from build123d import *

# Parameters (mm, degrees)
F1_DEPTH  = 30
F3_DEPTH  = 100
F4_R      = 50
F5_W      = 30
F5_H      = 30
F6_DEPTH  = 865
F8_W      = 1500
F8_H      = 460
F9_DEPTH  = 30
F11_W     = 780
F11_H     = 320
F12_DEPTH = 30
F13_W     = 30
F13_H     = 30
F14_DEPTH = 220
F15_W     = 30
F15_H     = 30
F16_DEPTH = 260
F17_W     = 780
F17_H     = 2
F18_DEPTH = 50
F19_R     = 20


with BuildPart() as f1:
    # F0 (on Top) → F1 (new body)
    with BuildSketch(Plane.XY):
        Polygon((0, 520), (0, 0), (1650, 0), (1650, 290), (1580, 290), (1580, 590), (150, 590), (150, 520), align=None)
    extrude(amount=F1_DEPTH)

    # F2 (on face) → F3 (join)
    with BuildSketch(Plane.XY.offset(30)):
        Polygon((1648, 0), (1650, 0), (1650, 290), (1580, 290), (1580, 590), (150, 590), (150, 520), (0, 520), (0, 518), (152, 518), (152, 588), (1578, 588), (1578, 288), (1648, 288), align=None)
    extrude(amount=F3_DEPTH)

    # F4
    f4_edges = [f1.edges().sort_by_distance(p)[0] for p in [
        (0, 519, 130),
        (1649, 0, 130),
    ]]
    fillet(f4_edges, radius=F4_R)

    # F5 (on face) → F6 (join)
    with BuildSketch(Plane(origin=(0, 0, 0), x_dir=(1, 0, 0), z_dir=(0, 0, -1))):
        with Locations((65, -45)):
            Rectangle(F5_W, F5_H)
        with Locations((1535, -45)):
            Rectangle(F5_W, F5_H)
        with Locations((1535, -475)):
            Rectangle(F5_W, F5_H)
        with Locations((65, -475)):
            Rectangle(F5_W, F5_H)
    extrude(amount=F6_DEPTH)

    # F8 (on offset) → F9 (join)
    with BuildSketch(Plane(origin=(0, 0, -715), x_dir=(1, 0, 0), z_dir=(0, 0, -1))):
        with Locations((800, -260)):
            Rectangle(F8_W, F8_H)
    extrude(amount=F9_DEPTH)



with BuildPart() as f12:
    # F11 (on offset) → F12 (new body)
    with BuildSketch(Plane.XY.offset(280)):
        with Locations((440, 185)):
            Rectangle(F11_W, F11_H)
    extrude(amount=-F12_DEPTH)


with BuildPart() as f1_1:
    add(f1.part)

    add(f12.part)  # F14 merges F12
    # F13 (on face) → F14 (join, through all)
    with BuildSketch(Plane(origin=(0, 0, 250), x_dir=(1, 0, 0), z_dir=(0, 0, -1))):
        with Locations((65, -40)):
            Rectangle(F13_W, F13_H)
        with Locations((65, -330)):
            Rectangle(F13_W, F13_H)
        with Locations((815, -40)):
            Rectangle(F13_W, F13_H)
        with Locations((815, -330)):
            Rectangle(F13_W, F13_H)
    extrude(amount=F14_DEPTH)

    # F15 (on face) → F16 (join, through all)
    with BuildSketch(Plane.XZ.offset(-315)):
        with Locations((65, 45)):
            Rectangle(F15_W, F15_H)
        with Locations((815, 45)):
            Rectangle(F15_W, F15_H)
    extrude(amount=F16_DEPTH)

    # F17 (on face) → F18 (join)
    with BuildSketch(Plane.XY.offset(280)):
        with Locations((440, 344)):
            Rectangle(F17_W, F17_H)
    extrude(amount=F18_DEPTH)

    # F19
    f19_edges = [f1_1.edges().sort_by_distance(p)[0] for p in [
        (50, 344, 330),
        (830, 344, 330),
    ]]
    fillet(f19_edges, radius=F19_R)


solid = f1_1.part
Check sheet for the modelled part. Datum: model origin and axes. Units: mm. A direction names the side the tool comes from. Round coordinates to 2 decimals unless told otherwise and drop trailing zeros. Loops run counter-clockwise (first coordinate to the right, second up) from the corner with the lowest first, then second, coordinate; pieces in that order, holes last. Notation, with made-up numbers: M -31,-36 L -17,-36 A21 ccw -17,-30 Z; hole C 24,17 d2. An arc over 180 degrees is marked long. One line per item, written item: value.
(1) Thickness scan on line 1 (Z direction, x = 471, y = 202); line 2 (X direction, y = 47.5, z = -491.5); line 3 (Z direction, x = 484, y = 407). Record the ranges inside material, lowest first.
Computed values:
line 1: z = -745 to -715, 0 to 30, 250 to 280
line 2: x = 50 to 80, 1520 to 1550
line 3: z = -745 to -715, 0 to 30
(2) Sectioned sample at B-B, the plane x = 1276.5. Record the cut outline in (y, z).
Computed values:
outline: M 0,0 L 590,0 L 590,130 L 588,130 L 588,30 L 0,30 Z; M 30,-745 L 490,-745 L 490,-715 L 30,-715 Z
(3) Sectioned sample at D-D, the plane x = 294. Record the cut outline in (y, z).
Computed values:
outline: M 0,0 L 590,0 L 590,130 L 588,130 L 588,30 L 0,30 Z; M 25,250 L 345,250 L 345,330 L 343,330 L 343,280 L 25,280 Z; M 30,-745 L 490,-745 L 490,-715 L 30,-715 Z
(4) Access from +Z, -Z, +X, -X, +Y, -Y to the whole of each face (thin tool, end or side, straight path). Record for faces 4 (the face through (1648, 146, 79)), 5 (the face through (438, 25, 257)), 6 (the face through (75, 518, 79)).
Computed values:
face 4: +Z, -Y
face 5: +Z, -X, -Y
face 6: +Z, -X
(5) Release check for a two-part mould opening along X. For faces 1 (the face through (76, 520, 64)), 2 (the face through (800, 186, 59)), 3 (the face through (50, 466, -463)) record: +X half, -X half, draft (parallel to the pull), parting line (faces both ways), or undercut.
Computed values:
face 1: draft
face 2: undercut
face 3: -X half
(6) Sectioned sample at A-A, the plane z = 188.5. Record the cut outline in (x, y).
Computed values:
outline: M 50,25 L 80,25 L 80,55 L 50,55 Z; M 50,315 L 80,315 L 80,345 L 50,345 Z; M 800,25 L 830,25 L 830,55 L 800,55 Z; M 800,315 L 830,315 L 830,345 L 800,345 Z
(7) Depth check by flat-ended pin: pin 1 Ø1.5 at (x, z) = (349, -728) entering from -Y; pin 2 Ø15 at (x, y) = (820.5, 136) entering from +Z; pin 3 Ø8 at (x, y) = (1228, 100.5) entering from +Z. Enter the tip coordinate at first touch or a pass-through.
Computed values:
pin 1: stops at y = 30
pin 2: stops at z = 280
pin 3: stops at z = 30
(8) Sectioned sample at C-C, the plane y = 371. Record the cut outline in (x, z).
Computed values:
outline: M 0,0 L 1580,0 L 1580,130 L 1578,130 L 1578,30 L 0,30 Z; M 50,-745 L 1550,-745 L 1550,-715 L 50,-715 Z
